Geometry: see drawing. Coordinates: mm, zero at the bounding-box minimum. A direction names the side the tool comes from. Coordinates: 2 decimals unless noted, no trailing zeros. Loops run counter-clockwise (first coordinate to the right, second up) from the corner with the lowest first, then second, coordinate; pieces in that order, holes last. Notation, with made-up numbers: (73, 54.5) - (108, 54.5) arc R16 cw to (108, 81.5) - close; hole circle Ø8 at (89.25, 84.5). An arc over 180 degrees is marked (long way). Use one line per item in the form item = value.
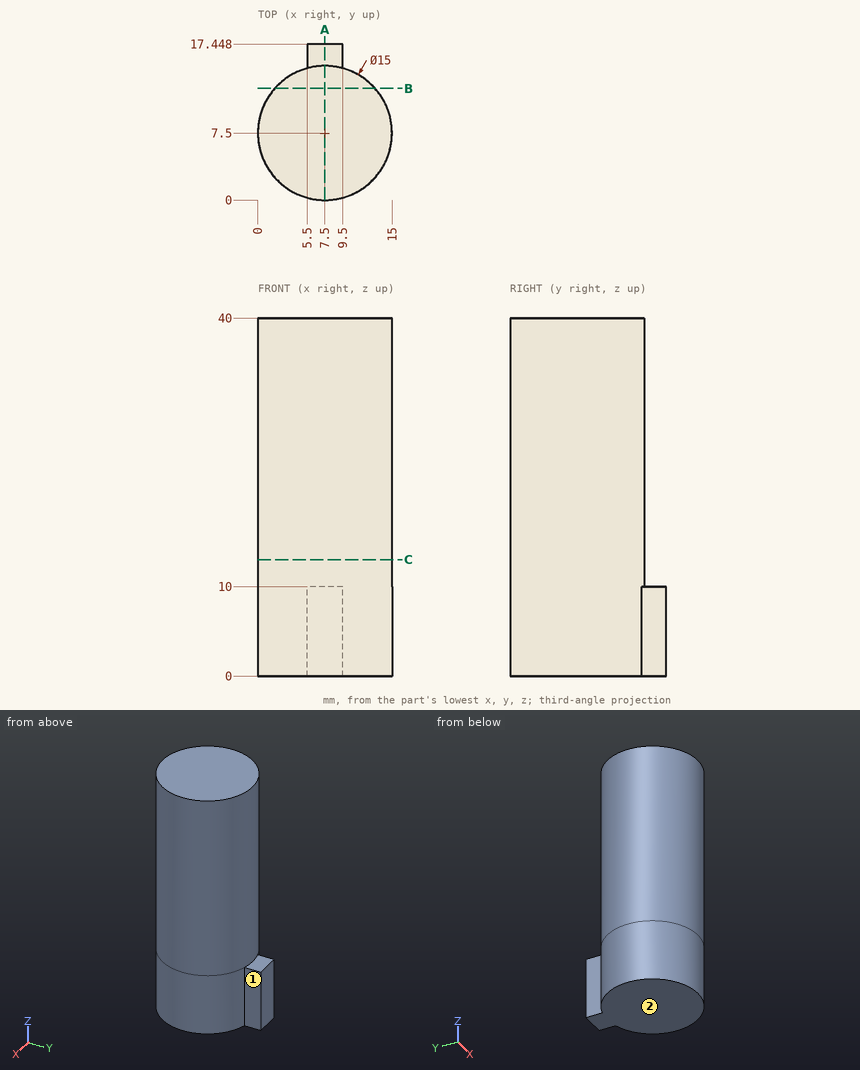
Q1. First-contact query: P1, Ø4, axis at y = 15, z = 34, coming from the +X side; P2, Ø1.5, axis at y = 12, z = 11, coming from the -X side (1 decimal); P3, Ø3, axis at y = 16.5, z = 6, coming from the -X side. Flat tips, straight axial feed; report the tip coordinate or a pass-through.
Check values:
P1 = 12.6
P2 = 1
P3 = 5.5
Q2. Ray query, line 1 along X through (y, z) = (4.25, 5.5); line 2 along Y through (x, z) = (12, 9.5); line 3 along X through (y, z) = (4, 32). Return the intervals inside material, ascending. Write a range as [from, to].
Check values:
line_1 = [0.74, 14.26]
line_2 = [1.5, 13.5]
line_3 = [0.87, 14.13]
Q3. Cut plane A-A, the plane x = 7.5. Return loops of the section in (y, z).
Check values:
outline = (0, 0) - (17.45, 0) - (17.45, 10) - (15, 10) - (15, 40) - (0, 40) - close
Q4. Set-up query: the marked faces 1 and 2. Return all of +Z, -Z, +X, -X, +Y, -Y with unobstructed straight access to the full face (end or side cutting, diameter ignored); none if empty.
Check values:
face_1 = +Z, -Z, +X, +Y
face_2 = -Z, +X, -X, +Y, -Y
Q5. Cut plane B-B, the plane y = 12.5. Return loops of the section in (x, z).
Check values:
outline = (1.91, 0) - (13.09, 0) - (13.09, 40) - (1.91, 40) - close
Q6. Cut plane C-C, the plane z = 13. Return loops of the section in (x, y), then the cut area to 3 significant figures.
Check values:
outline = circle Ø15 at (7.5, 7.5)
area = 177 mm²
